Input: part model. Units: mm. Frame: model coordinates. Face numbers are marked on the shaded views. A direction names the side the tool comes from. Coordinates: 2 decimals unless noted, no trailing zeros. Loops run counter-clockwise (first coordinate to the right, second up) from the corner with the lowest first, then second, coordinate; pieces in that order, holes last. Notation, with made-up numbers: (58, 27) -> (106, 27) arc R19 ccw to (106, 32) -> close; hole circle Ø2 at (17.5, 4). An arc over 180 degrees is marked (long way). Answer as a JSON object with one key per item and string values.
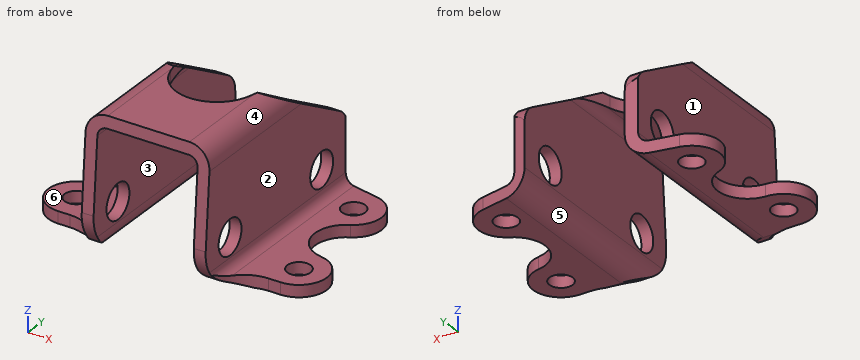
from build123d import *

# Parameters (mm, degrees)
F1_DEPTH = 25.4
F2_R     = 2.38125
F3_DEPTH = 12.7
F5_DEPTH = 63.5
F6_R     = 1.5875
F7_DEPTH = 63.5


with BuildPart() as f1:
    # F0 (on Front) → F1 (new body, symmetric)
    with BuildSketch(Plane.XZ):
        with BuildLine():
            Line((-33.1002511084, 1.6256), (-33.1002511084, 0))
            Line((-33.1002511084, 0), (-9.7536, 0))
            ThreePointArc((-9.7536, 0), (-7.7061016044, 0.8481016044), (-6.858, 2.8956))
            Line((-6.858, 2.8956), (-6.858, 16.1544))
            ThreePointArc((-6.858, 16.1544), (-6.4860256121, 17.0524256121), (-5.588, 17.4244))
            Line((-5.588, 17.4244), (5.588, 17.4244))
            ThreePointArc((5.588, 17.4244), (6.4860256121, 17.0524256121), (6.858, 16.1544))
            Line((6.858, 16.1544), (6.858, 2.8956))
            ThreePointArc((6.858, 2.8956), (7.7061016044, 0.8481016044), (9.7536, 0))
            Line((9.7536, 0), (35.6136485934, 0))
            Line((35.6136485934, 0), (35.6136485934, 1.6256))
            Line((35.6136485934, 1.6256), (9.7536, 1.6256))
            ThreePointArc((9.7536, 1.6256), (8.8555743879, 1.9975743879), (8.4836, 2.8956))
            Line((8.4836, 2.8956), (8.4836, 16.1544))
            ThreePointArc((8.4836, 16.1544), (7.6354983956, 18.2018983956), (5.588, 19.05))
            Line((5.588, 19.05), (-5.588, 19.05))
            ThreePointArc((-5.588, 19.05), (-7.6354983956, 18.2018983956), (-8.4836, 16.1544))
            Line((-8.4836, 16.1544), (-8.4836, 2.8956))
            ThreePointArc((-8.4836, 2.8956), (-8.8555743879, 1.9975743879), (-9.7536, 1.6256))
            Line((-9.7536, 1.6256), (-33.1002511084, 1.6256))
        make_face()
    extrude(amount=F1_DEPTH, both=True)

    # F2 (on Right) → F3 (cut, symmetric)
    with BuildSketch(Plane.YZ):
        with Locations((20.066, 5.588)):
            Circle(F2_R)
        with Locations((1.016, 5.588)):
            Circle(F2_R)
    extrude(amount=F3_DEPTH, both=True, mode=Mode.SUBTRACT)

    # F4 (on Right) → F5 (intersect, symmetric)
    with BuildSketch(Plane.YZ):
        with BuildLine():
            Line((-3.048, 19.05), (-4.0491707322, 5.9758729865))
            ThreePointArc((-4.0491707322, 5.9758729865), (-3.3726807453, 3.0295079996), (-1.142046819, 0.9891703742))
            Line((-1.142046819, 0.9891703742), (0.9658898494, 0))
            Line((0.9658898494, 0), (0.9658898494, -3.7190427538))
            Line((0.9658898494, -3.7190427538), (25.4, -3.7190427538))
            Line((25.4, -3.7190427538), (25.4, 0))
            Line((25.4, 0), (25.4, 8.763))
            ThreePointArc((25.4, 8.763), (24.9789926145, 10.3429207827), (23.8276222491, 11.5038441996))
            Line((23.8276222491, 11.5038441996), (10.922, 19.05))
            Line((10.922, 19.05), (-3.048, 19.05))
        make_face()
    extrude(amount=F5_DEPTH, both=True, mode=Mode.INTERSECT)

    # F6 (on Top) → F7 (intersect, symmetric)
    with BuildSketch(Plane.XY):
        with BuildLine():
            ThreePointArc((-14.0419021, 16.754134221), (-11.4555767164, 12.3367765251), (-15.24, 8.89))
            ThreePointArc((-15.24, 8.89), (-19.05, 5.08), (-15.24, 1.27))
            Line((-15.24, 1.27), (-13.5636, 1.27))
            ThreePointArc((-13.5636, 1.27), (-9.9714975516, -0.2178975516), (-8.4836, -3.81))
            Line((-8.4836, -3.81), (-8.4836, -8.5270870477))
            Line((-8.4836, -8.5270870477), (8.4836, -8.5270870477))
            Line((8.4836, -8.5270870477), (8.4836, -3.81))
            ThreePointArc((8.4836, -3.81), (9.9714975516, -0.2178975516), (13.5636, 1.27))
            Line((13.5636, 1.27), (15.24, 1.27))
            ThreePointArc((15.24, 1.27), (19.0391423785, 4.7925679424), (15.8132258851, 8.8466313975))
            ThreePointArc((15.8132258851, 8.8466313975), (12.203632925, 12.4056054875), (14.4638508851, 16.9428813975))
            ThreePointArc((14.4638508851, 16.9428813975), (16.4726911093, 20.8518851319), (13.4614256967, 24.0531395512))
            Line((13.4614256967, 24.0531395512), (6.858, 25.4))
            Line((6.858, 25.4), (6.858, 15.8741267216))
            add(Edge.make_bspline(
                [(6.7508981156, 15.0011278174), (6.858, 15.4184115393), (6.858, 15.8741267216)],
                knots=[4.2987589202, 4.2987589202, 4.2987589202, 4.7123889804, 4.7123889804, 4.7123889804], degree=2, weights=[1, 0.9786898915, 1]))
            Line((6.7508981156, 15.0011278174), (5.4125625526, 9.7867877722))
            ThreePointArc((5.4125625526, 9.7867877722), (0, 5.588), (-5.4125625526, 9.7867877722))
            Line((-5.4125625526, 9.7867877722), (-6.7508981156, 15.0011278174))
            Line((-6.7508981156, 15.0011278174), (-6.858, 15.4184115393))
            Line((-6.858, 15.4184115393), (-6.858, 15.8741267216))
            Line((-6.858, 15.8741267216), (-6.858, 25.4))
            Line((-6.858, 25.4), (-13.4614256967, 24.0531395512))
            ThreePointArc((-13.4614256967, 24.0531395512), (-16.4980082488, 20.6220485762), (-14.0419021, 16.754134221))
        make_face()
        with Locations((-15.24, 5.08)):
            Circle(F6_R, mode=Mode.SUBTRACT)
        with Locations((15.24, 5.08)):
            Circle(F6_R, mode=Mode.SUBTRACT)
        with Locations((-12.7, 20.32)):
            Circle(F6_R, mode=Mode.SUBTRACT)
        with Locations((12.7, 20.32)):
            Circle(F6_R, mode=Mode.SUBTRACT)
        with BuildLine():
            add(Edge.make_bspline(
                [(-6.858, 15.8741267216), (-6.858, 15.4184115393), (-6.7508981156, 15.0011278174)],
                knots=[1.5707963268, 1.5707963268, 1.5707963268, 1.984426387, 1.984426387, 1.984426387], degree=2, weights=[1, 0.9786898915, 1]))
            Line((-6.858, 15.8741267216), (-6.858, 15.4184115393))
            Line((-6.858, 15.4184115393), (-6.7508981156, 15.0011278174))
        make_face()
    extrude(amount=F7_DEPTH, both=True, mode=Mode.INTERSECT)


solid = f1.part
1. Mould query, pull axis X, two halves, no side actions, for the marked faces 4, 5 and 6. Classes: pulls with the +X half, pulls with the -X half, needs draft (parallel to the pull), parting line crosses it, or undercut.
Reply:
{"face 4": "pulls with the +X half", "face 5": "undercut", "face 6": "needs draft"}
2. Section query C-C (z = 14). Return loops of the section in (x, y), plus the area to 3 significant figures.
Reply:
{"outline": "(-8.48, -3.43) -> (-6.86, -3.43) -> (-6.86, 19.56) -> (-8.48, 19.56) -> close; (6.86, -3.43) -> (8.48, -3.43) -> (8.48, 19.56) -> (6.86, 19.56) -> close", "area": "74.8 mm2"}
3. Line query: line 1 along X through (y, z) = (4.25, 8.5); line 2 along X through (y, z) = (20.32, 0.6); line 3 along X through (y, z) = (20.32, 0.75). Output: solid intervals per line, ascending.
Reply:
{"line 1": "x = -8.48 to -6.86, 6.86 to 8.48", "line 2": "x = -16.51 to -14.29, -11.11 to -7.99, 7.99 to 11.11, 14.29 to 16.51", "line 3": "x = -16.51 to -14.29, -11.11 to -7.81, 7.81 to 11.11, 14.29 to 16.51"}
4. Section query D-D (z = 4.25). Return loops of the section in (x, y).
Reply:
{"outline": "(-8.48, -3.88) -> (-6.86, -3.88) -> (-6.86, -0.95) -> (-8.48, -0.95) -> close; (-8.48, 2.99) -> (-6.86, 2.99) -> (-6.86, 18.1) -> (-8.48, 18.1) -> close; (-8.48, 22.04) -> (-6.86, 22.04) -> (-6.86, 25.4) -> (-8.48, 25.07) -> close; (6.86, -3.88) -> (8.48, -3.88) -> (8.48, -0.95) -> (6.86, -0.95) -> close; (6.86, 2.99) -> (8.48, 2.99) -> (8.48, 18.1) -> (6.86, 18.1) -> close; (6.86, 22.04) -> (8.48, 22.04) -> (8.48, 25.07) -> (6.86, 25.4) -> close"}
5. Section query B-B (y = 4). Return loops of the section in (x, z), plus the area to 3 significant figures.
Reply:
{"outline": "(-18.89, 0) -> (-16.4, 0) -> (-16.4, 1.63) -> (-18.89, 1.63) -> close; (-14.08, 0) -> (-9.75, 0) arc R2.9 ccw to (-6.86, 2.9) -> (-6.86, 16.15) arc R1.27 cw to (-5.59, 17.42) -> (5.59, 17.42) arc R1.27 cw to (6.86, 16.15) -> (6.86, 2.9) arc R2.9 ccw to (9.75, 0) -> (14.08, 0) -> (14.08, 1.63) -> (9.75, 1.63) arc R1.27 cw to (8.48, 2.9) -> (8.48, 16.15) arc R2.9 ccw to (5.59, 19.05) -> (-5.59, 19.05) arc R2.9 ccw to (-8.48, 16.15) -> (-8.48, 2.9) arc R1.27 cw to (-9.75, 1.63) -> (-14.08, 1.63) -> close; (16.4, 0) -> (18.89, 0) -> (18.89, 1.63) -> (16.4, 1.63) -> close", "area": "105 mm2"}
6. Pin query (flat end, axial travel): P1, Ø10, axis at y = 16, z = 10, coming from the +X side; P2, Ø7.5, axis at y = 1.016, z = 5.588, coming from the -X side; P3, Ø1.9, axis at x = -12.7, y = 20.32, coming from the +Z side (3 decimals); P4, Ø0.8, axis at x = -14.5, z = 0.5, coming from the -Y side. Return the tip coordinate at first contact, or that it passes through.
Reply:
{"P1": "stops at x = 8.48", "P2": "stops at x = -9.05", "P3": "passes through", "P4": "stops at y = 1.27"}
7. Section query A-A (x = 12.7). Return loops of the section in (y, z).
Reply:
{"outline": "(1.2, 0) -> (11, 0) -> (11, 1.63) -> (1.2, 1.63) -> close; (15.23, 0) -> (18.73, 0) -> (18.73, 1.63) -> (15.23, 1.63) -> close; (21.91, 0) -> (24.21, 0) -> (24.21, 1.63) -> (21.91, 1.63) -> close"}
8. Access query for the marked faces 1, 2 and 3. Directions: +Z, -Z, +X, -X, +Y, -Y. A direction counts if a zero-diameter tool reaches every point of the face in a straight line with its end or side. Return the directions, or none.
Reply:
{"face 1": "+Z, -X, +Y, -Y", "face 2": "+Z, +X, +Y, -Y", "face 3": "-Z, +Y, -Y"}
